Can you work these out from the model? Positions are in its coordinate system, mm. Coordinates: 2 decimals unless noted, no trailing zeros. Order: outer loops, then holes, each group sorted by start corner. A loop starts at its lowest first (then second) coordinate and runs counter-clockwise, first axis right, second up. Notation, with made-up numbers: (79, -5.75) - (96, -5.75) arc R25 cw to (96, 22.25) - close; hole circle Ø8 at (-34, 63). An arc over 180 degrees is marked (long way). Return JSON: item names as keys, results as strings. Group by question number.
1) Imagine slicing it at B-B (y = 313.5). Write out the boundary of the cut face in (x, z).
2) For pin 1 Ø5 at (x, z) = (433, 15) entering from -Y; pin 2 Ø5.5 at (x, y) = (425, 351) entering from +Z; pin 3 Ø3 at (y, z) = (427, 3) entering from -X, each with a flat end and sliding along its axis, tell me the tip position at first contact or that it passes through.
3) Imagine slicing it at C-C (x = 309). Write out the boundary of the cut face in (y, z).
4) Imagine slicing it at D-D (y = 153). Write out the boundary of the cut face in (x, z), and give its area (3 significant figures).
5) If I drill on line 1 along X through (y, z) = (259.5, 14.25); line 2 along X through (y, z) = (22, 14.75); line 3 along Y through (x, z) = (-70, 6), over which ranges is the centre line in solid material (lowest first)?
6) Imagine slicing it at A-A (z = 14). Write out the boundary of the cut face in (x, y).
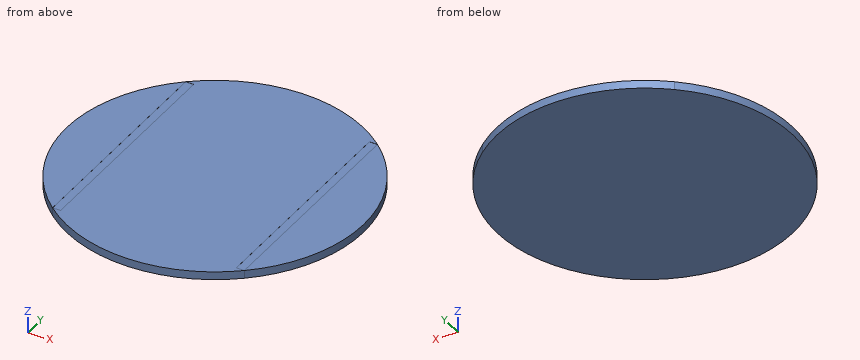
Autodesk Inventor part; units mm, degrees
ref_plane "YZ Plane" through (0, 0, 0) normal (1, 0, 0) x (0, 1, 0)
ref_plane "XZ Plane" through (0, 0, 0) normal (0, 1, 0) x (-1, 0, 0)
ref_plane "XY Plane" through (0, 0, 0) normal (0, 0, 1) x (1, 0, 0)
sketch "Sketch1" plane through (0, 0, 0) normal (0, 0, 1) x (1, 0, 0)
  line L0 (0, 0) -> (429.7172, 0)
  line L1 (429.7172, 0) -> (429.7172, 508)
  line L2 (429.7172, 508) -> (0, 508)
  line L3 (0, 508) -> (0, 0)
  line L4 (18.0086, 508) -> (18.0086, 0)
  line L5 (411.7086, 508) -> (411.7086, 0)
  circle A0 centre (214.8586, 254) radius 332.6864
  point P0 (0, 254)
  dimension "d1" = 508
  dimension "d3" = 18.0086
  dimension "d4" = 18.0086
  dimension "d6" = 393.7
  dimension "d10" = 665.3727
  dimension "d13" = 214.8586
  dimension "d14" = 254
extrude "Extrusion2" add sketch "Sketch1" along normal blind 18.0086 contours A0 L3 | L0 A0 | L4 L2 L5 L0 | A0 L2 | L1 A0
extrude "Extrusion3" add sketch "Sketch1" along normal blind 17.78 contours L3 L2 L4 L0 | L0 L5 L2 L1
properties part number "base turntable"
Calculated:
{
 "1": {"outline": "(-112.46, 0) - (542.18, 0) - (542.18, 18.01) - (429.72, 18.01) - (429.72, 17.78) - (411.71, 17.78) - (411.71, 18.01) - (18.01, 18.01) - (18.01, 17.78) - (0, 17.78) - (0, 18.01) - (-112.46, 18.01) - close"},
 "2": {"pin 1": "y = 0.66", "pin 2": "z = 17.78", "pin 3": "x = -70.22"},
 "3": {"outline": "(-65.09, 0) - (573.09, 0) - (573.09, 18.01) - (-65.09, 18.01) - close"},
 "4": {"outline": "(-102.13, 0) - (531.84, 0) - (531.84, 18.01) - (429.72, 18.01) - (429.72, 17.78) - (411.71, 17.78) - (411.71, 18.01) - (18.01, 18.01) - (18.01, 17.78) - (0, 17.78) - (0, 18.01) - (-102.13, 18.01) - close", "area": "11,400 mm2"},
 "5": {"line 1": "-117.78 to 547.5", "line 2": "-23.59 to 453.3", "line 3": "82.14 to 425.86"},
 "6": {"outline": "circle Ø665.37 at (214.86, 254)"}
}
